Can you work these out from the model? Positions are in its coordinate system, mm. A direction names the side the tool comes from. Coordinates: 2 decimals unless noted, no trailing zeros. Loops run counter-clockwise (first coordinate to the right, second up) from the corner with the lowest first, then second, coordinate; pieces in that order, holes last.
```python
from build123d import *

# Parameters (mm, degrees)
BASE_SKETCH_W       = 150
BASE_SKETCH_H       = 50
BASE_SKETCH_W_2     = 3.2
BASE_SKETCH_H_2     = 10
BOSS_EXTRUDE1_DEPTH = 3.2
FILLET1_R           = 10


with BuildPart() as part:
    # Base_Sketch → Boss-Extrude1 (new body)
    with BuildSketch(Plane(origin=(0, 0, 0), x_dir=(1, 0, 0), z_dir=(0, 1, 0))):
        Rectangle(BASE_SKETCH_W, BASE_SKETCH_H)
        with Locations((-25, 0)):
            Rectangle(BASE_SKETCH_W_2, BASE_SKETCH_H_2, mode=Mode.SUBTRACT)
    extrude(amount=BOSS_EXTRUDE1_DEPTH)

    # Fillet1
    fillet1_edges = [part.edges().sort_by_distance(p)[0] for p in [
        (75, 1.6, 25),
        (-75, 1.6, 25),
        (-75, 1.6, -25),
        (75, 1.6, -25),
    ]]
    fillet(fillet1_edges, radius=FILLET1_R)


solid = part.part
```
Item 1: Suppose I cut it at A-A, the plane y = 1.4. Please give me the cut outline in (x, z).
Results are:
outline: (-75, -15) arc R10 ccw to (-65, -25) - (65, -25) arc R10 ccw to (75, -15) - (75, 15) arc R10 ccw to (65, 25) - (-65, 25) arc R10 ccw to (-75, 15) - close; hole (-26.6, -5) - (-23.4, -5) - (-23.4, 5) - (-26.6, 5) - close
Item 2: On a 3-axis mill with a long thin cutter (end or side, diameter ignored), from which of +Z, -Z, +X, -X, +Y, -Y can I reach the whole of each face in a straight line? I mean faces 1 (the face through (-72.15, 1.62, 21.99)), 2 (the face through (-26.6, 2, 0)). Say none if no direction works.
Results are:
face 1: +Z, -X, +Y, -Y
face 2: +Y, -Y
Item 3: I need wall thicknesses on line 1 along X through (y, z) = (1.8, 3.5); line 2 along Z through (x, y) = (-25.5, 1.9); line 3 along X through (y, z) = (2.65, 15.5). Which ranges of each line are inside material? Lowest first, please.
Results are:
line 1: x = -75 to -26.6, -23.4 to 75
line 2: z = -25 to -5, 5 to 25
line 3: x = -74.99 to 74.99
Item 4: We'd pull the mould along Z, two halves only. Please class faces 3 (the face through (71.99, 1.62, 22.15)), 4 (the face through (-25, 2, -5)), 5 (the face through (-75, 2, 0)): +Z half, -Z half, draft (parallel to the pull), parting line (faces both ways), or undercut.
Results are:
face 3: +Z half
face 4: undercut
face 5: draft
Item 5: Suppose I cut it at B-B, the plane z = 22.5. Please give me the cut outline in (x, y).
Results are:
outline: (-71.61, 0) - (71.61, 0) - (71.61, 3.2) - (-71.61, 3.2) - close
